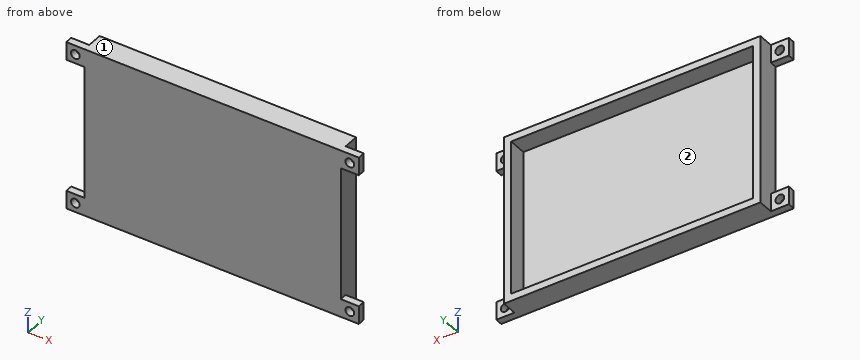
```python
from build123d import *

# Parameters (mm, degrees)
SKETCH1_W           = 90.17
SKETCH1_H           = 59.69
SKETCH1_W_2         = 85.09
SKETCH1_H_2         = 54.61
BOSS_EXTRUDE1_DEPTH = 6.35
SKETCH2_W           = 90.17
SKETCH2_H           = 59.69
BOSS_EXTRUDE2_DEPTH = 1.5875
SKETCH3_W           = 6.35
SKETCH3_H           = 6.35
SKETCH3_R           = 1.55
BOSS_EXTRUDE3_DEPTH = 2.54


with BuildPart() as part:
    # Sketch1 → Boss-Extrude1 (new body)
    with BuildSketch(Plane(origin=(0, 0, 0), x_dir=(1, 0, 0), z_dir=(0, 1, 0))):
        with Locations((42.545, 27.305)):
            Rectangle(SKETCH1_W, SKETCH1_H)
        with Locations((42.545, 27.305)):
            Rectangle(SKETCH1_W_2, SKETCH1_H_2, mode=Mode.SUBTRACT)
    extrude(amount=BOSS_EXTRUDE1_DEPTH)

    # Sketch2 → Boss-Extrude2 (add)
    with BuildSketch(Plane.XZ):
        with Locations((42.545, -27.305)):
            Rectangle(SKETCH2_W, SKETCH2_H)
    extrude(amount=BOSS_EXTRUDE2_DEPTH)

    # Sketch3 → Boss-Extrude3 (add)
    # profile 1 of 4: a face of its own
    with BuildSketch(Plane.XZ.offset(1.5875)):
        with Locations((90.805, -0.635)):
            Rectangle(SKETCH3_W, SKETCH3_H)
        with Locations(Location((90.805, -0.635, 0), (0, 0, 270))):
            Circle(SKETCH3_R, mode=Mode.SUBTRACT)
    # profile 2 of 4: a face of its own
    with BuildSketch(Plane.XZ.offset(1.5875)):
        with Locations((-5.715, -0.635)):
            Rectangle(SKETCH3_W, SKETCH3_H)
        with Locations(Location((-5.715, -0.635, 0), (0, 0, 270))):
            Circle(SKETCH3_R, mode=Mode.SUBTRACT)
    # profile 3 of 4: a face of its own
    with BuildSketch(Plane.XZ.offset(1.5875)):
        with Locations((-5.715, -53.975)):
            Rectangle(SKETCH3_W, SKETCH3_H)
        with Locations(Location((-5.715, -53.975, 0), (0, 0, 270))):
            Circle(SKETCH3_R, mode=Mode.SUBTRACT)
    # profile 4 of 4: a face of its own
    with BuildSketch(Plane.XZ.offset(1.5875)):
        with Locations((90.805, -53.975)):
            Rectangle(SKETCH3_W, SKETCH3_H)
        with Locations(Location((90.805, -53.975, 0), (0, 0, 270))):
            Circle(SKETCH3_R, mode=Mode.SUBTRACT)
    extrude(amount=-BOSS_EXTRUDE3_DEPTH)


solid = part.part
```
CAD build for the part. Positions are in the model's coordinates, mm. Face numbers are marked on the shaded views. Coordinates: 2 decimals unless noted, no trailing zeros. Write each loop counter-clockwise with the first axis right and the second up, starting at its lowest first coordinate (ties: lowest second). Pieces come first, ordered by that corner, then holes. Notation, with made-up numbers: (-16, 6) -> (17, 6) arc R16 ccw to (17, 14) -> close; hole circle Ø2 at (-39, 31.5). An arc over 180 degrees is marked (long way). Return JSON: item names as keys, results as strings. Group by question number.
Q1. Cut at A-A, the plane y = 5. Give the cut face in (x, z).
Q2. Flat gauge pins, fed straight in: pin 1 (1.9 mm diameter, centred on x = -5.715, z = -53.975, fed in from -Y); pin 2 (3.5 mm diameter, centred on x = 90.805, z = -53.975, fed in from +Y); pin 3 (2 mm diameter, centred on y = 2.5, z = -15.5, fed in from -X); pin 4 (1 mm diameter, centred on x = 20, z = -40, fed in from +Y). Where does each tip first touch, or does it go through?
Q3. Drill centre lines: line 1 (X direction, y = 1.75, z = -22.5); line 2 (Z direction, x = 39.5, y = 2.75); line 3 (X direction, y = -0.5, z = -1). Where is each one in solid material? Low to high.
Q4. Cut at C-C, the plane z = -32.5. Give the cut face in (x, y), then the cut area to 3 significant figures.
Q5. Cut at B-B, the plane x = 84. Give the cut face in (y, z).
Q6. Pull direction X, two halves, no side cores. Call the marked faces 1 and 2: released by +X, released by -X, zero draft, split by the parting line, or undercut.
Returned:
{
 "1": {"outline": "(-2.54, -57.15) -> (87.63, -57.15) -> (87.63, 2.54) -> (-2.54, 2.54) -> close; hole (0, -54.61) -> (85.09, -54.61) -> (85.09, 0) -> (0, 0) -> close"},
 "2": {"pin 1": "passes through", "pin 2": "stops at y = 0.95", "pin 3": "stops at x = -2.54", "pin 4": "stops at y = 0"},
 "3": {"line 1": "x = -2.54 to 0, 85.09 to 87.63", "line 2": "z = -57.15 to -54.61, 0 to 2.54", "line 3": "x = -8.89 to -7.22, -4.21 to 89.3, 92.31 to 93.98"},
 "4": {"outline": "(-2.54, -1.59) -> (87.63, -1.59) -> (87.63, 6.35) -> (85.09, 6.35) -> (85.09, 0) -> (0, 0) -> (0, 6.35) -> (-2.54, 6.35) -> close", "area": "175 mm2"},
 "5": {"outline": "(-1.59, -57.15) -> (6.35, -57.15) -> (6.35, -54.61) -> (0, -54.61) -> (0, 0) -> (6.35, 0) -> (6.35, 2.54) -> (-1.59, 2.54) -> close"},
 "6": {"face 1": "zero draft", "face 2": "undercut"}
}
